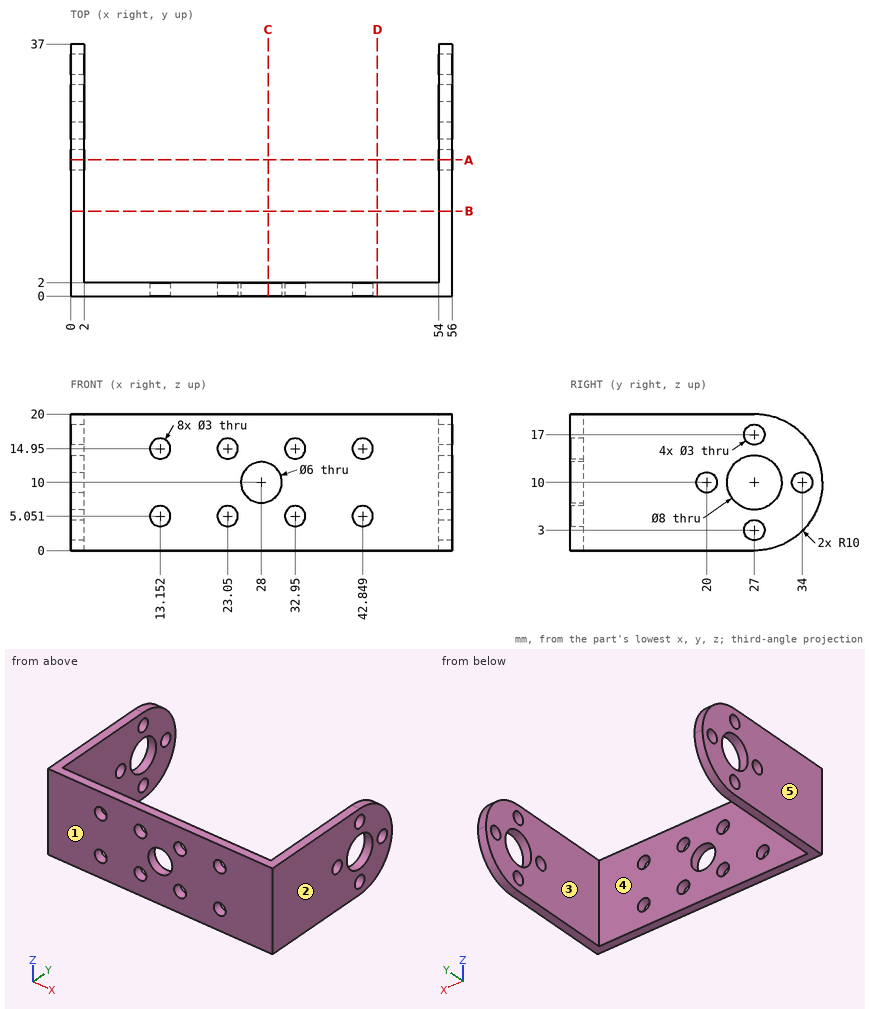
Design review of the part shown in the three views and the two pictorial views. Dimensions are in mm from the part's minimum x, y and z. A direction names the side the tool comes from. Round coordinates to 2 decimals unless told otherwise and drop trailing zeros. Write each loop counter-clockwise with the first axis right and the second up, starting at its lowest first coordinate (ties: lowest second). Pieces come first, ordered by that corner, then holes. Notation, with made-up numbers: (-27, 39) -> (19, 39) arc R21 cw to (19, 51) -> close; hole circle Ø1 at (-39.75, -19.75). An arc over 180 degrees is marked (long way). Answer as a JSON object with one key per item and string values.
1. The part is to be moulded in two halves that separate along X. For the marked faces 1, 2 and 3, say which applies: pulls with the +X half, pulls with the -X half, needs draft (parallel to the pull), parting line crosses it, or undercut.
Results found:
{"face 1": "needs draft", "face 2": "pulls with the +X half", "face 3": "undercut"}
2. We need section D-D on x = 45. State the section outline as (y, z) points, and give its area (3 significant figures).
Results found:
{"outline": "(0, 0) -> (2, 0) -> (2, 20) -> (0, 20) -> close", "area": "40.0 mm^2"}
3. To check wall thickness, follow line 1 along Y through (x, z) = (54.65, 10); line 2 along X through (y, z) = (35, 7.75); line 3 along Y through (x, z) = (27, 16.75). State the ranges of each line that lie inside material, in increasing order.
Results found:
{"line 1": "y = 0 to 18.5, 21.5 to 23, 31 to 32.5, 35.5 to 37", "line 2": "x = 0 to 2, 54 to 56", "line 3": "y = 0 to 2"}
4. Machinability: for the marked faces 4 and 5, which of the approach directions +Z, -Z, +X, -X, +Y, -Y give a long, thin tool a straight path to every point of the face, cutting with its end or side? Answer none if there is none.
Results found:
{"face 4": "+Z, -Z, +Y", "face 5": "+Z, -Z, -X, +Y, -Y"}
5. Clearance check with flat-ended pins moving along their axes: pin 1 (2.5 mm diameter, centred on x = 23.05, z = 5.05, fed in from +Y); pin 2 (3.5 mm diameter, centred on y = 27, z = 3, fed in from -X); pin 3 (4 mm diameter, centred on x = 14.5, z = 3, fed in from +Y). State where each tip first meets the part, or that it passes through.
Results found:
{"pin 1": "passes through", "pin 2": "stops at x = 0", "pin 3": "stops at y = 2"}
6. We need section A-A on y = 20. State the section outline as (x, z) points.
Results found:
{"outline": "(0, 0) -> (2, 0) -> (2, 8.5) -> (0, 8.5) -> close; (0, 11.5) -> (2, 11.5) -> (2, 20) -> (0, 20) -> close; (54, 0) -> (56, 0) -> (56, 8.5) -> (54, 8.5) -> close; (54, 11.5) -> (56, 11.5) -> (56, 20) -> (54, 20) -> close"}
7. We need section B-B on y = 12.5. State the section outline as (x, z) points.
Results found:
{"outline": "(0, 0) -> (2, 0) -> (2, 20) -> (0, 20) -> close; (54, 0) -> (56, 0) -> (56, 20) -> (54, 20) -> close"}
8. We need section C-C on x = 29. State the section outline as (y, z) points.
Results found:
{"outline": "(0, 0) -> (2, 0) -> (2, 7.17) -> (0, 7.17) -> close; (0, 12.83) -> (2, 12.83) -> (2, 20) -> (0, 20) -> close"}
